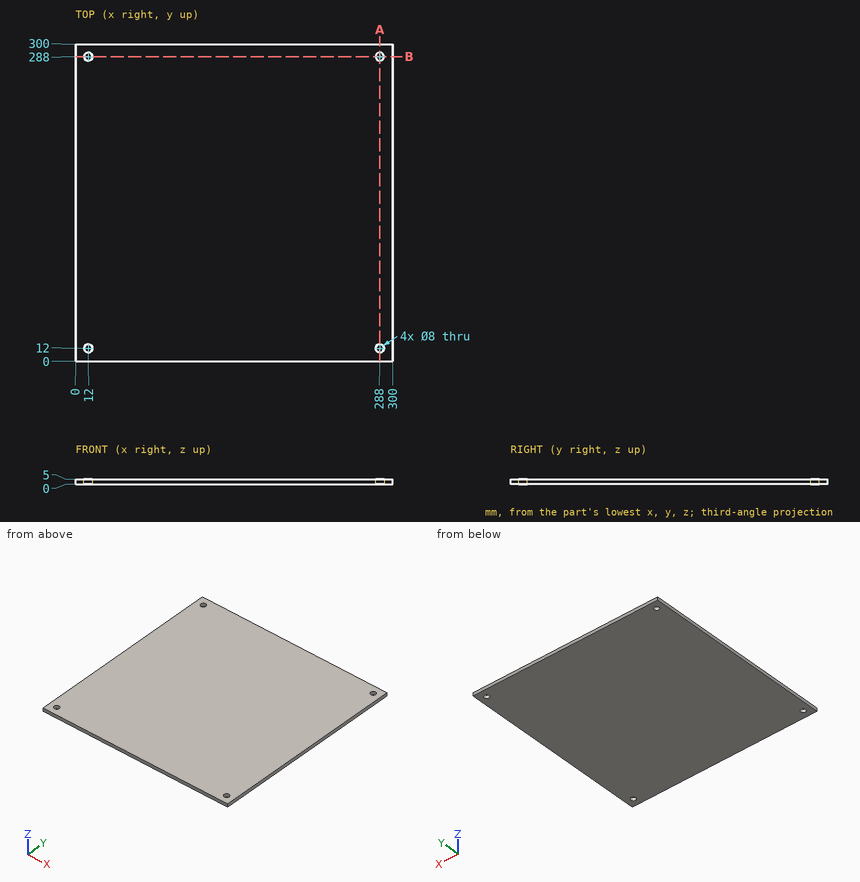
Drawing for the job (mm, zero at the part's lowest x, y, z). Round coordinates to 2 decimals unless told otherwise and drop trailing zeros. Write each loop counter-clockwise with the first axis right and the second up, starting at its lowest first coordinate (ties: lowest second). Pieces come first, ordered by that corner, then holes. Notation, with made-up numbers: M -14.75,-16.75 L -4.75,-16.75 A19 cw -4.75,3.25 Z; hole C 8.5,84 d1. An arc over 180 degrees is marked long. Answer as a JSON object with one key per item and string values. Group by question number.
(1) Drill centre line: L1, parallel to Y at x = 288, z = 2. Where is it in solid material? Low to high.
(2) Cut at A-A (x = 288). Give the cut face in (y, z), and give its area (3 significant figures).
(3) Flat gauge pins, fed straight in: pin 1 (1.5 mm diameter, centred on y = 226.5, z = 0.5, fed in from -X); pin 2 (6.5 mm diameter, centred on x = 288, y = 12, fed in from +Z) (1 decimal). Where does each tip first touch, or does it go through?
Responses:
{
 "1": {"L1": "y = 0 to 8, 16 to 284, 292 to 300"},
 "2": {"outline": "M 0,0 L 8,0 L 8,5 L 0,5 Z; M 16,0 L 284,0 L 284,5 L 16,5 Z; M 292,0 L 300,0 L 300,5 L 292,5 Z", "area": "1,420 mm2"},
 "3": {"pin 1": "stops at x = 0", "pin 2": "passes through"}
}
